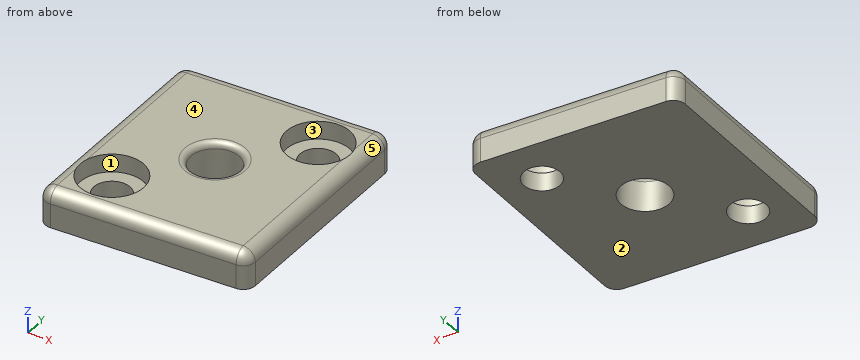
from build123d import *

# Parameters (mm, degrees)
F0_R         = 1.5
F0_R_2       = 2
F1_DEPTH     = 3
F2_R         = 2.625
F2_R_2       = 1.5
F3_DEPTH     = 1.5
F4_T1_DEPTH  = 4.3472443006
F4_T3_DEPTH  = 16.2344954865
F4_T5_DEPTH  = 14.8006020278
F4_T7_DEPTH  = 4.6626968477
F4_T9_DEPTH  = 16.2344954865
F4_T11_DEPTH = 14.8006020278
F4_T16_DEPTH = 1
F4_T22_DEPTH = 1
F4_T28_DEPTH = 1
F4_T34_DEPTH = 1
F5_R         = 0.5


# Not quite as in the source:
# - a fillet or chamfer that OpenCascade refuses, or shapes differently, is made with other operations: its cross-section is extruded or revolved along the edge and cut away or added


with BuildPart() as f1:
    # F0 (on Top) → F1 (new body)
    with BuildSketch(Plane.XY):
        Polygon((8.4645454874, -8.5124193832), (8.2962074114, 9.7252756798), (-8.4645454874, 8.5124193832), (-8.2962074114, -9.7252756798), align=None)
        with Locations((-4.8033426305, -5.6307453454)):
            Circle(F0_R, mode=Mode.SUBTRACT)
        Polygon((4.02705255, 0.3354530665), (2.3040371523, -3.3198032774), (-1.7230153977, -3.6552563439), (-4.02705255, -0.3354530665), (-2.3040371523, 3.3198032774), (1.7230153977, 3.6552563439), align=None, mode=Mode.SUBTRACT)
        with Locations((4.8033426305, 5.6307453454)):
            Circle(F0_R, mode=Mode.SUBTRACT)
        Polygon((-1.7230153977, -3.6552563439), (2.3040371523, -3.3198032774), (4.02705255, 0.3354530665), (1.7230153977, 3.6552563439), (-2.3040371523, 3.3198032774), (-4.02705255, -0.3354530665), align=None)
        Circle(F0_R_2, mode=Mode.SUBTRACT)
    extrude(amount=F1_DEPTH)

    # F2 (on face) → F3 (cut)
    with BuildSketch(Plane.XY.offset(3)):
        with Locations((-4.8033426305, -5.6307453454)):
            Circle(F2_R)
        with Locations((-4.8033426305, -5.6307453454)):
            Circle(F2_R_2, mode=Mode.SUBTRACT)
        with Locations((4.8033426305, 5.6307453454)):
            Circle(F2_R)
        with Locations((4.8033426305, 5.6307453454)):
            Circle(F2_R_2, mode=Mode.SUBTRACT)
    extrude(amount=-F3_DEPTH, mode=Mode.SUBTRACT)

    # F4: fillet of radius 1 on 8 edges, made by hand

    # F4_s2 → F4_t1 (cut)
    with BuildSketch(Plane.XY.offset(-2.3472443006)):
        with BuildLine():
            ThreePointArc((-7.5280963703, 8.5801835352), (-8.1912373991, 8.2605167863), (-8.4558796169, 7.573561656))
            Line((-8.4558796169, 7.573561656), (-8.4645454874, 8.5124193832))
            Line((-8.4645454874, 8.5124193832), (-7.5280963703, 8.5801835352))
        make_face()
        with BuildLine():
            ThreePointArc((8.4558796169, -7.573561656), (8.1912373991, -8.2605167863), (7.5280963703, -8.5801835352))
            Line((7.5280963703, -8.5801835352), (8.4645454874, -8.5124193832))
            Line((8.4645454874, -8.5124193832), (8.4558796169, -7.573561656))
        make_face()
    extrude(amount=F4_T1_DEPTH, mode=Mode.SUBTRACT)

    # F4_s4 → F4_t3 (cut)
    with BuildSketch(Plane(origin=(-0.0706200975, 7.6509595097, 0), x_dir=(0, 0, 1), z_dir=(0.0092298344, -0.9999574042, 0))):
        with BuildLine():
            ThreePointArc((3, 7.3856167117), (2.7071067812, 8.0927234929), (2, 8.3856167117))
            Line((2, 8.3856167117), (3, 8.3856167117))
            Line((3, 8.3856167117), (3, 7.3856167117))
        make_face()
    extrude(amount=F4_T3_DEPTH, mode=Mode.SUBTRACT)

    # F4_s6 → F4_t5 (cut)
    with BuildSketch(Plane(origin=(7.8907735218, 0.570999072, 0), x_dir=(0, 0, 1), z_dir=(-0.9973920448, -0.0721741576, 0))):
        with BuildLine():
            ThreePointArc((2, 9.1011408148), (2.7071067812, 8.808247596), (3, 8.1011408148))
            Line((3, 8.1011408148), (3, 9.1011408148))
            Line((3, 9.1011408148), (2, 9.1011408148))
        make_face()
    extrude(amount=F4_T5_DEPTH, mode=Mode.SUBTRACT)

    # F4_s8 → F4_t7 (cut)
    with BuildSketch(Plane.XY.offset(-2.6626968477)):
        with BuildLine():
            ThreePointArc((8.3060379118, 8.6602423087), (7.9838058035, 9.3863276607), (7.23390635, 9.648404519))
            Line((7.23390635, 9.648404519), (8.2962074114, 9.7252756798))
            Line((8.2962074114, 9.7252756798), (8.3060379118, 8.6602423087))
        make_face()
        with BuildLine():
            ThreePointArc((-7.23390635, -9.648404519), (-7.9838058035, -9.3863276607), (-8.3060379118, -8.6602423087))
            Line((-8.3060379118, -8.6602423087), (-8.2962074114, -9.7252756798))
            Line((-8.2962074114, -9.7252756798), (-7.23390635, -9.648404519))
        make_face()
    extrude(amount=F4_T7_DEPTH, mode=Mode.SUBTRACT)

    # F4_s10 → F4_t9 (cut)
    with BuildSketch(Plane(origin=(0.0706200975, -7.6509595097, 0), x_dir=(0, 0, 1), z_dir=(-0.0092298344, 0.9999574042, 0))):
        with BuildLine():
            ThreePointArc((2, 8.3856167117), (2.7071067812, 8.0927234929), (3, 7.3856167117))
            Line((3, 7.3856167117), (3, 8.3856167117))
            Line((3, 8.3856167117), (2, 8.3856167117))
        make_face()
    extrude(amount=F4_T9_DEPTH, mode=Mode.SUBTRACT)

    # F4_s12 → F4_t11 (cut)
    with BuildSketch(Plane(origin=(-7.8907735218, -0.570999072, 0), x_dir=(0, 0, 1), z_dir=(0.9973920448, 0.0721741576, 0))):
        with BuildLine():
            ThreePointArc((2, 9.1011408148), (2.7071067812, 8.808247596), (3, 8.1011408148))
            Line((3, 8.1011408148), (3, 9.1011408148))
            Line((3, 9.1011408148), (2, 9.1011408148))
        make_face()
    extrude(amount=F4_T11_DEPTH, mode=Mode.SUBTRACT)


with BuildPart() as f4_tool14:
    # F4_s15 → F4_t16 (new body)
    with BuildSketch(Plane.XY.offset(2)):
        Polygon((-7.4559222127, 7.5827914904), (-8.4558796169, 7.573561656), (-8.4645454874, 8.5124193832), (-7.5280963703, 8.5801835352), align=None)
    extrude(amount=F4_T16_DEPTH)

    # F4_s17 → F4_t18 (revolve, cut)
    with BuildSketch(Plane(origin=(-7.4559222127, 7.5827914904, 2), x_dir=(0.7353151864, -0.6777252959, 0), z_dir=(-0.6777252959, -0.7353151864, 0))):
        with BuildLine():
            ThreePointArc((0, -1), (1, 0), (0, 1))
            Line((0, 1), (0, -1))
        make_face()
    revolve(axis=Axis((-7.4559222127, 7.5827914904, 2), (0, 0, 1)), mode=Mode.SUBTRACT)


with BuildPart() as f1_1:
    add(f1.part)

    # F4_t13: cut F4_tool14
    add(f4_tool14.part, mode=Mode.SUBTRACT)


with BuildPart() as f4_tool20:
    # F4_s21 → F4_t22 (new body)
    with BuildSketch(Plane.XY.offset(2)):
        Polygon((-7.3060805076, -8.6510124742), (-8.3060379118, -8.6602423087), (-8.2962074114, -9.7252756798), (-7.23390635, -9.648404519), align=None)
    extrude(amount=F4_T22_DEPTH)

    # F4_s23 → F4_t24 (revolve, cut)
    with BuildSketch(Plane(origin=(-7.3060805076, -8.6510124742, 2), x_dir=(0.6777252959, 0.7353151864, 0), z_dir=(0.7353151864, -0.6777252959, 0))):
        with BuildLine():
            ThreePointArc((0, -1), (1, 0), (0, 1))
            Line((0, 1), (0, -1))
        make_face()
    revolve(axis=Axis((-7.3060805076, -8.6510124742, 2), (0, 0, 1)), mode=Mode.SUBTRACT)


with BuildPart() as f1_2:
    add(f1_1.part)

    # F4_t19: cut F4_tool20
    add(f4_tool20.part, mode=Mode.SUBTRACT)


with BuildPart() as f4_tool26:
    # F4_s27 → F4_t28 (new body)
    with BuildSketch(Plane.XY.offset(2)):
        Polygon((7.3060805076, 8.6510124742), (8.3060379118, 8.6602423087), (8.2962074114, 9.7252756798), (7.23390635, 9.648404519), align=None)
    extrude(amount=F4_T28_DEPTH)

    # F4_s29 → F4_t30 (revolve, cut)
    with BuildSketch(Plane(origin=(7.3060805076, 8.6510124742, 2), x_dir=(-0.6777252959, -0.7353151864, 0), z_dir=(-0.7353151864, 0.6777252959, 0))):
        with BuildLine():
            ThreePointArc((0, -1), (1, 0), (0, 1))
            Line((0, 1), (0, -1))
        make_face()
    revolve(axis=Axis((7.3060805076, 8.6510124742, 2), (0, 0, 1)), mode=Mode.SUBTRACT)


with BuildPart() as f1_3:
    add(f1_2.part)

    # F4_t25: cut F4_tool26
    add(f4_tool26.part, mode=Mode.SUBTRACT)


with BuildPart() as f4_tool32:
    # F4_s33 → F4_t34 (new body)
    with BuildSketch(Plane.XY.offset(2)):
        Polygon((7.4559222127, -7.5827914904), (8.4558796169, -7.573561656), (8.4645454874, -8.5124193832), (7.5280963703, -8.5801835352), align=None)
    extrude(amount=F4_T34_DEPTH)

    # F4_s35 → F4_t36 (revolve, cut)
    with BuildSketch(Plane(origin=(7.4559222127, -7.5827914904, 2), x_dir=(-0.7353151864, 0.6777252959, 0), z_dir=(0.6777252959, 0.7353151864, 0))):
        with BuildLine():
            ThreePointArc((0, -1), (1, 0), (0, 1))
            Line((0, 1), (0, -1))
        make_face()
    revolve(axis=Axis((7.4559222127, -7.5827914904, 2), (0, 0, 1)), mode=Mode.SUBTRACT)


with BuildPart() as f1_4:
    add(f1_3.part)

    # F4_t31: cut F4_tool32
    add(f4_tool32.part, mode=Mode.SUBTRACT)

    # F5
    f5_edges = [f1_4.edges().sort_by_distance(p)[0] for p in [
        (-2, 0, 3),
    ]]
    fillet(f5_edges, radius=F5_R)


solid = f1_4.part
The listing builds one solid part. Answer for the finished solid, in the listing's coordinates (mm). Face numbers are marked on the shaded views. A direction names the side the tool comes from. Give positions to 0.01 mm unless a question says otherwise; leave off trailing zeros. Write each loop counter-clockwise with the first axis right and the second up, starting at its lowest first coordinate (ties: lowest second). Pieces come first, ordered by that corner, then holes. Notation, with made-up numbers: (79.5, 30) -> (134.5, 30) arc R28 ccw to (134.5, 69) -> close; hole circle Ø6 at (-4, 9.5). An arc over 180 degrees is marked (long way). One line per question, with ' | ' between items. Start each with the question number.
1. For the marked faces 1 and 2, determine the directions among +Z, -Z, +X, -X, +Y, -Y from which every point of the face is accessible in a straight line to the end or side of a thin tool.
2. Find the intervals of material crossed by probe 1 along Z at (x, y) = (7.5, -6); probe 2 along Y at (x, z) = (-7, 1.75); probe 3 along Y at (x, z) = (-1.75, 0.3), in increasing order.
3. Given pin 1 Ø5 at (x, y) = (0.5, -3.5) entering from -Z; pin 2 Ø1.6 at (x, y) = (-5, -7) entering from +Z, each flat-ended and moving along its own axis, determine where each tip first touches the part or whether it passes through.
4. For a pull along X with two mould halves and no side action, classify the marked faces 3, 4 and 5 as pulls with the +X half, pulls with the -X half, needs draft (parallel to the pull), parting line crosses it, or undercut.
5. Section A-A (z = 0.65) is taken. Determine the outline of the cut face in (x, y), plus the area to 3 significant figures.
Response values:
1) face 1: +Z | face 2: -Z, +X, -X, +Y, -Y
2) probe 1: 0 to 3 | probe 2: -9.63 to -7.07, -4.19 to 8.62 | probe 3: -9.25 to -0.97, 0.97 to 9
3) pin 1: z = 0 | pin 2: z = 1.5
4) face 3: undercut | face 4: needs draft | face 5: pulls with the +X half
5) outline: (-8.46, 7.57) -> (-8.31, -8.66) arc R1 ccw to (-7.23, -9.65) -> (7.53, -8.58) arc R1 ccw to (8.46, -7.57) -> (8.31, 8.66) arc R1 ccw to (7.23, 9.65) -> (-7.53, 8.58) arc R1 ccw to start; hole circle Ø3 at (-4.8, -5.63); hole circle Ø4 at (0, 0); hole circle Ø3 at (4.8, 5.63) | area: 278 mm2
